Here's how the part is built. I have some questions about the finished solid (model axes, mm). Face numbers are marked on the shaded views. Round coordinates to 2 decimals unless told otherwise and drop trailing zeros. Loops run counter-clockwise (first coordinate to the right, second up) from the corner with the lowest first, then second, coordinate; pieces in that order, holes last. Notation, with made-up numbers: M -35,6 L 15,6 A15 cw 15,12 Z; hole C 83,-11.5 d11. An arc over 180 degrees is marked long. Use a Markdown table: item, result.
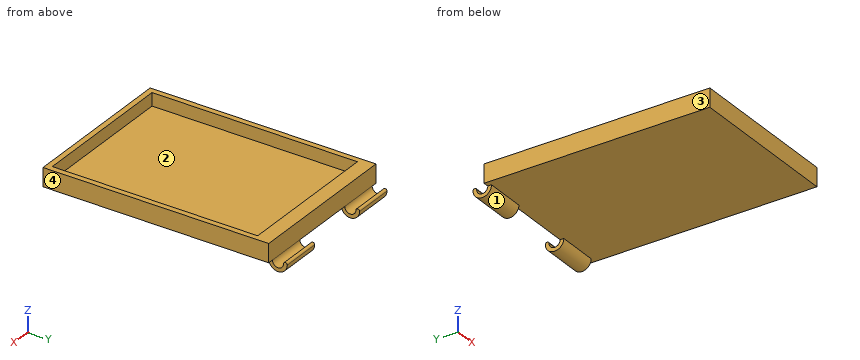
```python
from build123d import *

# Parameters (mm, degrees)
EKRAN_TABAN_W               = 86
EKRAN_TABAN_H               = 117
EKRAN_TABAN_W_2             = 80
EKRAN_TABAN_H_2             = 111
Y_KSEKLIK_EKSTR_ZYON1_DEPTH = 10
EKRAN_TABAN_2_W             = 80
EKRAN_TABAN_2_H             = 111
Y_KSEKLIK_EKSTR_ZYON2_DEPTH = 3
Y_KSEKLIK_EKSTR_ZYON3_DEPTH = 86
IZIM6_W                     = 3
IZIM6_H                     = 15
IZIM6_W_2                   = 36
KES_EKSTR_ZYON3_DEPTH       = 10
IZIM8_W                     = 3
IZIM8_H                     = 5
IZIM8_W_2                   = 36
KES_EKSTR_ZYON5_DEPTH       = 2


with BuildPart() as part:
    # ekran_taban → Yükseklik-Ekstrüzyon1 (new body)
    with BuildSketch(Plane.XY):
        with Locations((2.953774531, 19.102589183)):
            Rectangle(EKRAN_TABAN_W, EKRAN_TABAN_H)
        with Locations((2.953774531, 19.102589183)):
            Rectangle(EKRAN_TABAN_W_2, EKRAN_TABAN_H_2, mode=Mode.SUBTRACT)
    extrude(amount=Y_KSEKLIK_EKSTR_ZYON1_DEPTH)

    # ekran_taban<2> → Yükseklik-Ekstrüzyon2 (add)
    with BuildSketch(Plane.XY):
        with Locations((2.953774531, 19.102589183)):
            Rectangle(EKRAN_TABAN_2_W, EKRAN_TABAN_2_H)
    extrude(amount=Y_KSEKLIK_EKSTR_ZYON2_DEPTH)

    # Çizim3 → Yükseklik-Ekstrüzyon3 (add)
    with BuildSketch(Plane(origin=(45.953774531, 0, 0), x_dir=(0, 0, -1), z_dir=(1, 0, 0))):
        with BuildLine():
            Line((-10, 77.602589183), (0, 77.602589183))
            Line((0, 77.602589183), (0, 80.602589183))
            ThreePointArc((0, 80.602589183), (5, 85.602589183), (0, 90.602589183))
            ThreePointArc((0, 90.602589183), (-1, 89.602589183), (0, 88.602589183))
            ThreePointArc((0, 88.602589183), (3, 85.602589183), (0, 82.602589183))
            Line((0, 82.602589183), (-10, 82.602589183))
            Line((-10, 82.602589183), (-10, 77.602589183))
        make_face()
    extrude(amount=-Y_KSEKLIK_EKSTR_ZYON3_DEPTH)

    # Çizim6 → Kes-Ekstrüzyon3 (cut)
    with BuildSketch(Plane(origin=(0, 82.602589183, 0), x_dir=(1, 0, 0), z_dir=(0, 1, 0))):
        with Locations((-38.546225469, -2.5)):
            Rectangle(IZIM6_W, IZIM6_H)
        with Locations((2.953774531, -2.5)):
            Rectangle(IZIM6_W_2, IZIM6_H)
        with Locations((44.453774531, -2.5)):
            Rectangle(IZIM6_W, IZIM6_H)
    extrude(amount=KES_EKSTR_ZYON3_DEPTH, mode=Mode.SUBTRACT)

    # Çizim8 → Kes-Ekstrüzyon5 (cut)
    with BuildSketch(Plane(origin=(0, 82.602589183, 0), x_dir=(1, 0, 0), z_dir=(0, 1, 0))):
        with Locations((-38.546225469, 2.5)):
            Rectangle(IZIM8_W, IZIM8_H)
        with Locations((44.453774531, 2.5)):
            Rectangle(IZIM8_W, IZIM8_H)
        with Locations((2.953774531, 2.5)):
            Rectangle(IZIM8_W_2, IZIM8_H)
    extrude(amount=-KES_EKSTR_ZYON5_DEPTH, mode=Mode.SUBTRACT)


solid = part.part
```
Q1. We'd pull the mould along X, two halves only. Please class the marked faces 1, 2, 3 and 4: pulls with the +X half, pulls with the -X half, needs draft (parallel to the pull), parting line crosses it, or undercut.
Return value:
| item | result |
|---|---|
| face 1 | needs draft |
| face 2 | undercut |
| face 3 | pulls with the -X half |
| face 4 | pulls with the +X half |
Q2. Imagine slicing it at A-A, the plane x = 38. Please give me the cut outline in (y, z).
Return value:
| item | result |
|---|---|
| outline | M -39.4,0 L 80.6,0 A5 ccw 90.6,0 A1 ccw 88.6,0 A3 cw 82.6,0 L 82.6,10 L 74.6,10 L 74.6,3 L -36.4,3 L -36.4,10 L -39.4,10 Z |
Q3. Imagine slicing it at B-B, the plane y = 5. Please give me the cut outline in (x, z).
Return value:
| item | result |
|---|---|
| outline | M -40.05,0 L 45.95,0 L 45.95,10 L 42.95,10 L 42.95,3 L -37.05,3 L -37.05,10 L -40.05,10 Z |
Q4. Will these pins go through, and if not, where does the flat tip stop? P1, Ø5.5, axis at x = 22.5, z = 6.5, coming from the +Y side; P2, Ø2, axis at x = -25, y = 19.5, coming from the -Z side; P3, Ø1, axis at x = 28.5, z = -3.5, coming from the -Y side; P4, Ø1.8, axis at y = 87.5, z = -0.5, coming from the +X side.
Return value:
| item | result |
|---|---|
| P1 | stops at y = 82.6 |
| P2 | stops at z = 0 |
| P3 | stops at y = 81.6 |
| P4 | passes through |
Q5. I need wall thicknesses on line 1 (Y direction, x = -12.5, z = 3.75); line 2 (X direction, y = 12, z = 4); line 3 (Z direction, x = -3, y = 46.5). Which ranges of each line are inside material? Lowest first, please. Write a range as from..to.
Return value:
| item | result |
|---|---|
| line 1 | y = -39.4..-36.4, 74.6..82.6 |
| line 2 | x = -40.05..-37.05, 42.95..45.95 |
| line 3 | z = 0..3 |
